Build history of the part. All positions in model axes, mm. Face numbers are marked on the shaded views. A direction names the side the tool comes from. Round coordinates to 2 decimals unless told otherwise and drop trailing zeros. Write each loop counter-clockwise with the first axis right and the second up, starting at its lowest first coordinate (ties: lowest second). Pieces come first, ordered by that corner, then holes.
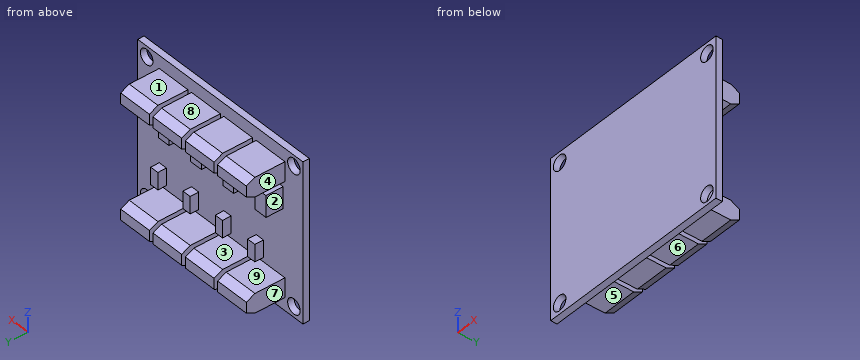
from build123d import *

# Parameters (mm, degrees)
SKETCH1_W           = 46
SKETCH1_H           = 37
SKETCH1_R           = 1.75
BOSS_EXTRUDE1_DEPTH = 0.75
SKETCH2_W           = 8
SKETCH2_H           = 4.5
BOSS_EXTRUDE2_DEPTH = 9
CUT_EXTRUDE2_DEPTH  = 124
SKETCH4_W           = 2
SKETCH4_H           = 4
BOSS_EXTRUDE3_DEPTH = 2
SKETCH5_W           = 3
SKETCH5_H           = 5
BOSS_EXTRUDE4_DEPTH = 4


with BuildPart() as part:
    # Sketch1 → Boss-Extrude1 (new, symmetric)
    with BuildSketch(Plane(origin=(0, 0, 0), x_dir=(1, 0, 0), z_dir=(0, 1, 0))):
        Rectangle(SKETCH1_W, SKETCH1_H)
        with Locations(Location((20.5, 16, 0), (0, 0, 270))):
            Circle(SKETCH1_R, mode=Mode.SUBTRACT)
        with Locations(Location((20.5, -16, 0), (0, 0, 90))):
            Circle(SKETCH1_R, mode=Mode.SUBTRACT)
        with Locations(Location((-20.5, -16, 0), (0, 0, 270))):
            Circle(SKETCH1_R, mode=Mode.SUBTRACT)
        with Locations(Location((-20.5, 16, 0), (0, 0, 90))):
            Circle(SKETCH1_R, mode=Mode.SUBTRACT)
    extrude(amount=BOSS_EXTRUDE1_DEPTH, both=True)

    # Sketch2 → Boss-Extrude2 (add)
    with BuildSketch(Plane(origin=(0, 0.75, 0), x_dir=(1, 0, 0), z_dir=(0, 1, 0))):
        with Locations((13, 13.25)):
            Rectangle(SKETCH2_W, SKETCH2_H)
        with Locations((4, 13.25)):
            Rectangle(SKETCH2_W, SKETCH2_H)
        with Locations((-5, 13.25)):
            Rectangle(SKETCH2_W, SKETCH2_H)
        with Locations((-14, 13.25)):
            Rectangle(SKETCH2_W, SKETCH2_H)
        with Locations((-14, -13.25)):
            Rectangle(SKETCH2_W, SKETCH2_H)
        with Locations((-5, -13.25)):
            Rectangle(SKETCH2_W, SKETCH2_H)
        with Locations((4, -13.25)):
            Rectangle(SKETCH2_W, SKETCH2_H)
        with Locations((13, -13.25)):
            Rectangle(SKETCH2_W, SKETCH2_H)
    extrude(amount=BOSS_EXTRUDE2_DEPTH)

    # Sketch3 → Cut-Extrude2 (cut)
    with BuildSketch(Plane(origin=(17, 0, 0), x_dir=(0, 0, -1), z_dir=(1, 0, 0))):
        Polygon((-15.5, 9.75), (-15.5, 7.75), (-14.5, 9.75), align=None)
        Polygon((-11, 9.75), (-12, 9.75), (-11, 7.75), align=None)
        Polygon((12, 9.75), (11, 9.75), (11, 7.75), align=None)
        Polygon((15.5, 7.75), (14.5, 9.75), (15.5, 9.75), align=None)
    extrude(amount=-CUT_EXTRUDE2_DEPTH, mode=Mode.SUBTRACT)

    # Sketch4 → Boss-Extrude3 (add)
    with BuildSketch(Plane(origin=(0, 0.75, 0), x_dir=(1, 0, 0), z_dir=(0, 1, 0))):
        with Locations((16, 8)):
            Rectangle(SKETCH4_W, SKETCH4_H)
        with Locations((7, 8)):
            Rectangle(SKETCH4_W, SKETCH4_H)
        with Locations((-2, 8)):
            Rectangle(SKETCH4_W, SKETCH4_H)
        with Locations((-11, 8)):
            Rectangle(SKETCH4_W, SKETCH4_H)
    extrude(amount=BOSS_EXTRUDE3_DEPTH)

    # Sketch5 → Boss-Extrude4 (add)
    with BuildSketch(Plane(origin=(0, 0.75, 0), x_dir=(1, 0, 0), z_dir=(0, 1, 0))):
        with Locations((-16, -7)):
            Rectangle(SKETCH5_W, SKETCH5_H)
        with Locations((-7, -7)):
            Rectangle(SKETCH5_W, SKETCH5_H)
        with Locations((2, -7)):
            Rectangle(SKETCH5_W, SKETCH5_H)
        with Locations((11, -7)):
            Rectangle(SKETCH5_W, SKETCH5_H)
    extrude(amount=BOSS_EXTRUDE4_DEPTH)


solid = part.part
1) Which spindle directions (+Z, -Z, +X, -X, +Y, -Y) get a long thin tool onto all of the face, cutting with end or side? Do the marked faces 1, 2, 3, 4 and 5. Say none if no direction does.
Results:
face 1: +Z, +X, -X, +Y
face 2: -X, +Y
face 3: +X, -X, +Y
face 4: +Z, -Z, -X, +Y
face 5: -Z, +X, -X, +Y
2) Slice it at A-A (z = 16). Write the cut outline in (x, y), plus the area to 3 significant figures.
Results:
outline: (-23, -0.75) - (-22.25, -0.75) - (-22.25, 0.75) - (-23, 0.75) - close; (-18.75, -0.75) - (18.75, -0.75) - (18.75, 0.75) - (-18.75, 0.75) - close; (22.25, -0.75) - (23, -0.75) - (23, 0.75) - (22.25, 0.75) - close
area: 58.5 mm2
3) Slice it at D-D (x = -14). Write the cut outline in (y, z), plus the area to 4 significant figures.
Results:
outline: (-0.75, -18.5) - (0.75, -18.5) - (0.75, -15.5) - (7.75, -15.5) - (9.75, -14.5) - (9.75, -12) - (7.75, -11) - (0.75, -11) - (0.75, 11) - (7.75, 11) - (9.75, 12) - (9.75, 14.5) - (7.75, 15.5) - (0.75, 15.5) - (0.75, 18.5) - (-0.75, 18.5) - close
area: 132.5 mm2
4) Slice it at C-C (x = 20.5). Write the cut outline in (y, z).
Results:
outline: (-0.75, -18.5) - (0.75, -18.5) - (0.75, -17.75) - (-0.75, -17.75) - close; (-0.75, -14.25) - (0.75, -14.25) - (0.75, 14.25) - (-0.75, 14.25) - close; (-0.75, 17.75) - (0.75, 17.75) - (0.75, 18.5) - (-0.75, 18.5) - close
5) Wall check: L1, parallel to Z at x = 16.5, y = 2; L2, parallel to Z at x = 1, y = 4; L3, parallel to X at y = 0.3, z = -16. Give the ranges that are in metal, low to high.
Results:
L1: z = -15.5 to -11, -10 to -6, 11 to 15.5
L2: z = -15.5 to -11, 4.5 to 9.5, 11 to 15.5
L3: x = -23 to -22.25, -18.75 to 18.75, 22.25 to 23
6) Slice it at B-B (y = 5.5). Count the separate pieces of the cut face and the enclosed holes in it, plus the area to 3 significant figures.
Results:
separate pieces: 8
enclosed holes: 0
area: 288 mm2
7) Pin check, flat tips, straight feed: pin 1 Ø0.9 at (x, y) = (-7.5, 2) entering from -Z; pin 2 Ø2 at (x, y) = (-10, 7) entering from +Z; pin 3 Ø5 at (y, z) = (4.5, -5) entering from +X. Stop position of each tip, or through.
Results:
pin 1: stops at z = -15.5
pin 2: stops at z = 15.5
pin 3: stops at x = 17
8) Mould opens along Z. For the marked faces 6, 7, 8 and 9 say: released by +Z, released by -Z, zero draft, split by the parting line, or undercut.
Results:
face 6: released by -Z
face 7: zero draft
face 8: released by +Z
face 9: undercut
